Read the model definition and answer for the solid it produces. Units are mm, in the model's axes. A direction names the side the tool comes from. Round coordinates to 2 decimals unless told otherwise and drop trailing zeros. Order: outer loops, then holes, each group sorted by start corner. A loop starts at its lowest first (then second) coordinate and runs counter-clockwise, first axis right, second up.
from build123d import *

# Parameters (mm, degrees)
SKETCH1_R           = 12
SKETCH1_R_2         = 7.5
BOSS_EXTRUDE1_DEPTH = 14
SKETCH6_R           = 17.5
SKETCH6_R_2         = 12
BOSS_EXTRUDE4_DEPTH = 21
BOSS_EXTRUDE5_DEPTH = 9
CUT_EXTRUDE4_DEPTH  = 6.5


with BuildPart() as part:
    # Sketch1 → Boss-Extrude1 (new body, symmetric)
    with BuildSketch(Plane(origin=(0, 0, 0), x_dir=(1, 0, 0), z_dir=(0, 1, 0))):
        Circle(SKETCH1_R)
        Circle(SKETCH1_R_2, mode=Mode.SUBTRACT)
    extrude(amount=BOSS_EXTRUDE1_DEPTH, both=True)



with BuildPart() as body_2:
    # Sketch6 → Boss-Extrude4 (new body, symmetric)
    with BuildSketch(Plane(origin=(0, 0, 0), x_dir=(1, 0, 0), z_dir=(0, 1, 0))):
        with Locations((178, 0)):
            Circle(SKETCH6_R)
        with Locations((178, 0)):
            Circle(SKETCH6_R_2, mode=Mode.SUBTRACT)
    extrude(amount=BOSS_EXTRUDE4_DEPTH, both=True)


with BuildPart() as part_1:
    add(part.part)

    add(body_2.part)  # Boss-Extrude5 merges body 2
    # Sketch14 → Boss-Extrude5 (add, symmetric)
    with BuildSketch(Plane(origin=(0, 0, 0), x_dir=(1, 0, 0), z_dir=(0, 1, 0))):
        with BuildLine():
            Line((7.937253933, -9), (162.99166898, -9))
            ThreePointArc((162.99166898, -9), (160.5, 0), (162.99166898, 9))
            Line((162.99166898, 9), (7.937253933, 9))
            ThreePointArc((7.937253933, 9), (12, 0), (7.937253933, -9))
        make_face()
    extrude(amount=BOSS_EXTRUDE5_DEPTH, both=True)

    # Sketch16 → Cut-Extrude4 (cut)
    with BuildSketch(Plane(origin=(0, 9, 0), x_dir=(1, 0, 0), z_dir=(0, 1, 0))):
        with BuildLine():
            Line((20, 5), (150, 5))
            ThreePointArc((150, 5), (155, 0), (150, -5))
            Line((150, -5), (20, -5))
            ThreePointArc((20, -5), (15, 0), (20, 5))
        make_face()
    cut_extrude4 = extrude(amount=-CUT_EXTRUDE4_DEPTH, mode=Mode.SUBTRACT)

    # Mirror1: Cut-Extrude4 across plane
    add(cut_extrude4.mirror(Plane.ZX), mode=Mode.SUBTRACT)


solid = part_1.part
Q1. For faces 3 (the face through (87, 0, -9)), 4 (the face through (86, -6, 5)), 5 (the face through (84, 0, 9)), 6 (the face through (86, 6, 5)), determine the directions among +Z, -Z, +X, -X, +Y, -Y from which every point of the face is accessible in a straight line to the end or side of a thin tool.
Outcome:
face 3: -Z, +Y, -Y
face 4: -Y
face 5: +Z, +Y, -Y
face 6: +Y
Q2. A cutting plane is placed at C-C, the plane z = 0. Give the vertices of the cut face in (x, y).
Outcome:
outline: (-12, -14) - (-7.5, -14) - (-7.5, 14) - (-12, 14) - close; (7.5, -14) - (12, -14) - (12, -9) - (15, -9) - (15, -2.5) - (155, -2.5) - (155, -9) - (160.5, -9) - (160.5, -21) - (166, -21) - (166, 21) - (160.5, 21) - (160.5, 9) - (155, 9) - (155, 2.5) - (15, 2.5) - (15, 9) - (12, 9) - (12, 14) - (7.5, 14) - close; (190, -21) - (195.5, -21) - (195.5, 21) - (190, 21) - close
Q3. Straight lines are drawn through the part: probe 1 along X at (y, z) = (5, 0); probe 2 along Z at (x, y) = (178, -3); probe 3 along X at (y, z) = (0, 3). For each, find the intervals that lie inside material, in ascending order.
Outcome:
probe 1: x = -12 to -7.5, 7.5 to 15, 155 to 166, 190 to 195.5
probe 2: z = -17.5 to -12, 12 to 17.5
probe 3: x = -11.62 to -6.87, 6.87 to 166.38, 189.62 to 195.24
Q4. Flat-ended cylindrical pins translate along their axes: pin 1 (14.5 mm diameter, centred on x = 109.5, z = 4, fed in from -Y); pin 2 (12 mm diameter, centred on x = 104, z = -11, fed in from +Y); pin 3 (12 mm diameter, centred on y = 6, z = -8, fed in from +X). Find the tip coordinate at first contact, or state that the pin passes through.
Outcome:
pin 1: stops at y = -9
pin 2: stops at y = 9
pin 3: stops at x = 195.39
Q5. A cutting plane is placed at B-B, the plane x = 0. Give the vertices of the cut face in (y, z), plus the area to 3 significant figures.
Outcome:
outline: (-14, -12) - (14, -12) - (14, -7.5) - (-14, -7.5) - close; (-14, 7.5) - (14, 7.5) - (14, 12) - (-14, 12) - close
area: 252 mm2
Q6. For a pull along X with two mould halves and no side action, classify faces 1 (the face through (15, 6, 0)), 2 (the face through (182, -21, -12)) as released by +X, released by -X, zero draft, split by the parting line, or undercut.
Outcome:
face 1: undercut
face 2: zero draft
Q7. A cutting plane is placed at D-D, the plane x = 77. Give the vertices of the cut face in (y, z).
Outcome:
outline: (-9, -9) - (9, -9) - (9, -5) - (2.5, -5) - (2.5, 5) - (9, 5) - (9, 9) - (-9, 9) - (-9, 5) - (-2.5, 5) - (-2.5, -5) - (-9, -5) - close
Q8. A cutting plane is placed at A-A, the plane y = -7. Give the vertices of the cut face in (x, z).
Outcome:
outline: (7.94, -9) - (162.99, -9) arc R17.5 ccw (long way) to (162.99, 9) - (7.94, 9) arc R12 ccw (long way) to start; hole circle Ø15 at (0, 0); hole (20, -5) - (150, -5) arc R5 ccw to (150, 5) - (20, 5) arc R5 ccw to start; hole circle Ø24 at (178, 0)
